Work out the finished part from the listing and answer in its coordinate system (mm). A direction names the side the tool comes from. Give positions to 0.01 mm unless a question says otherwise; leave off trailing zeros. Loops run counter-clockwise (first coordinate to the right, second up) from the corner with the lowest first, then second, coordinate; pieces in that order, holes last. Notation, with made-up numbers: (25, 71) - (82, 71) arc R24 cw to (82, 87) - close; hole circle Ø4 at (69, 10). An arc over 180 degrees is marked (long way). One line per item, written item: value.
from build123d import *
from build123d.topology import SkipClean

# Parameters (mm, degrees)
BOSS_EXTRUDE3_DEPTH = 1


with BuildPart() as part:
    # Sketch1 → Revolve2 (revolve)
    with BuildSketch(Plane.XY, mode=Mode.PRIVATE) as revolve2_sk:
        Polygon((0, 0), (31.5, 0), (31.5, 1.75), (6.25, 2.25), (6.25, 2.63), (0, 2.75), align=None)
    revolve(revolve2_sk.sketch.rotate(Axis((0, 0, 0), (1, 0, 0)), 90), axis=Axis((0, 0, 0), (1, 0, 0)))

    # Sketch3 → Boss-Extrude3 (add, symmetric)
    with BuildSketch(Plane.XY):
        with BuildLine():
            Line((31.5, 1.75), (34.86, 1.683465347))
            ThreePointArc((34.86, 1.683465347), (36.252723474, 0), (34.86, -1.683465347))
            Line((34.86, -1.683465347), (31.5, -1.75))
            Line((31.5, -1.75), (31.5, 1.75))
        make_face()
    extrude(amount=BOSS_EXTRUDE3_DEPTH, both=True)

    # Sketch9 → Cut-Revolve9 (revolve, cut)
    with SkipClean():  # the faces are left unmerged after this step: merging them gives an invalid solid
        with BuildSketch(Plane.XY):
            Polygon((31.5, 1.75), (31.5, 2.5), (37.130328502, 2.5), (37.130328502, 1.638508346), align=None)
        revolve(axis=Axis((31.5, 0, 0), (1, 0, 0)), mode=Mode.SUBTRACT)

    # Sketch7 → Cut-Revolve8 (revolve, cut)
    with SkipClean():  # the faces are left unmerged after this step: merging them gives an invalid solid
        with BuildSketch(Plane.XY):
            Polygon((31.5, 1.75), (31.5, 2.588823056), (36.825315724, 2.588823056), (36.825315724, 1.644548203), align=None)
        revolve(axis=Axis((31.5, 0, 0), (1, 0, 0)), mode=Mode.SUBTRACT)


solid = part.part
1. For faces 1 (the flat face through (34, 0, 1)), 2 (the conical face through (3.1, -1.8, -2)), 3 (the flat face through (34, 0, -1)), determine the directions among +Z, -Z, +X, -X, +Y, -Y from which every point of the face is accessible in a straight line to the end or side of a thin tool.
Output:
face 1: +Z, +X, +Y, -Y
face 2: +X
face 3: -Z, +X, +Y, -Y
2. Flat-ended cylindrical pins translate along their axes: pin 1 Ø2.5 at (x, y) = (35, 0) entering from +Z; pin 2 Ø0.8 at (y, z) = (-0.5, 1.5) entering from +X; pin 3 Ø1.4 at (x, y) = (34, 0) entering from -Z. Find the tip coordinate at first contact, or state that the pin passes through.
Output:
pin 1: stops at z = 1
pin 2: stops at x = 31.5
pin 3: stops at z = -1
3. Section B-B (x = 25.5) is taken. Write down the section's boundary in (y, z).
Output:
outline: circle Ø3.74 at (0, 0)
4. Section A-A (x = 21.5) is taken. Write down the section's boundary in (y, z).
Output:
outline: circle Ø3.9 at (0, 0)
5. Find the intervals of material crossed by line 1 along X through (y, z) = (1.3, -2); line 2 along X through (y, z) = (-0.65, 1.2); line 3 along Z through (x, y) = (24, 0.6), in increasing order.
Output:
line 1: x = 0 to 6.25
line 2: x = 0 to 31.5
line 3: z = -1.8 to 1.8
